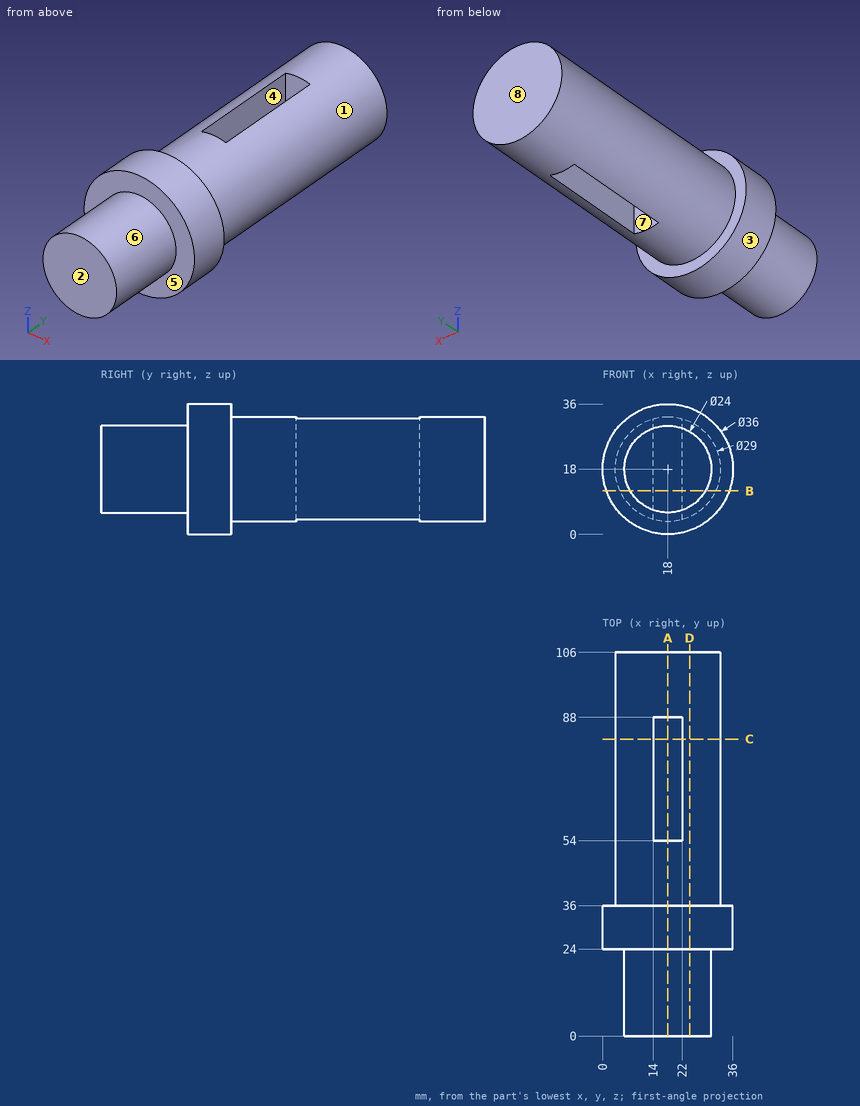
Can you work these out from the drawing? Everything is in mm from the part's minimum corner. A direction names the side the tool comes from. Give positions to 0.01 mm unless a question says otherwise; leave off trailing zeros. Order: outer loops, then holes, each group sorted by start corner. A loop starts at its lowest first (then second) coordinate and runs counter-clockwise, first axis right, second up.
Item 1: I'm going to push flat-ended pins straight in: pin 1 (12 mm diameter, centred on x = 31.5, y = 61.5, fed in from +Z); pin 2 (4 mm diameter, centred on x = 14, y = 19.5, fed in from +Z); pin 3 (9 mm diameter, centred on x = 20, z = 13, fed in from -Y); pin 4 (6 mm diameter, centred on y = 47.5, z = 29, fed in from -X). Where does each tip first touch, or does it pass through?
Item 2: If we section it at B-B, the plane z = 12: Write out the boundary of the cut face in (x, y).
Item 3: If we section it at C-C, the plane y = 82: Write out the boundary of the cut face in (x, z).
Item 4: For the marked faces 1, 2, 3, 4 and 5, which set-ups out of +Z, -Z, +X, -X, +Y, -Y let a thin tool reach every point of the face, with its end or its side?
Item 5: I need wall thicknesses on line 1 (Y direction, x = 20, z = 6); line 2 (Y direction, x = 20, z = 11); line 3 (X direction, y = 86, z = 22). Which ranges of each line are inside material? Lowest first, please.
Item 6: If we section it at A-A, the plane x = 18: Write out the boundary of the cut face in (y, z), plus the area to 3 significant figures.
Item 7: If we mould it in two halves opening along X, with no side actions, what happens to the marked faces 6, 7 and 8? For each: pulls with the +X half, pulls with the -X half, needs draft (parallel to the pull), parting line crosses it, or undercut.
Item 8: If we section it at D-D, the plane x = 24: Write out the boundary of the cut face in (y, z).
Values:
1. pin 1: stops at z = 30.41
1. pin 2: stops at z = 29.83
1. pin 3: stops at y = 0
1. pin 4: stops at x = 5.91
2. outline: (1.03, 24) - (7.61, 24) - (7.61, 0) - (28.39, 0) - (28.39, 24) - (34.97, 24) - (34.97, 36) - (31.2, 36) - (31.2, 106) - (4.8, 106) - (4.8, 36) - (1.03, 36) - close; hole (14, 54) - (22, 54) - (22, 88) - (14, 88) - close
3. outline: (14, 4.06) - (14, 31.94) arc R14.5 ccw to start; (22, 4.06) arc R14.5 ccw to (22, 31.94) - close
4. face 1: +Y
4. face 2: +Z, -Z, +X, -X, -Y
4. face 3: +Y, -Y
4. face 4: +Z, -Z
4. face 5: -Y
5. line 1: y = 24 to 54, 88 to 106
5. line 2: y = 0 to 54, 88 to 106
5. line 3: x = 4.06 to 14, 22 to 31.94
6. outline: (0, 6) - (24, 6) - (24, 0) - (36, 0) - (36, 3.5) - (54, 3.5) - (54, 32.5) - (36, 32.5) - (36, 36) - (24, 36) - (24, 30) - (0, 30) - close; (88, 3.5) - (106, 3.5) - (106, 32.5) - (88, 32.5) - close
6. area: 2,050 mm2
7. face 6: parting line crosses it
7. face 7: undercut
7. face 8: needs draft
8. outline: (0, 7.61) - (24, 7.61) - (24, 1.03) - (36, 1.03) - (36, 4.8) - (106, 4.8) - (106, 31.2) - (36, 31.2) - (36, 34.97) - (24, 34.97) - (24, 28.39) - (0, 28.39) - close
